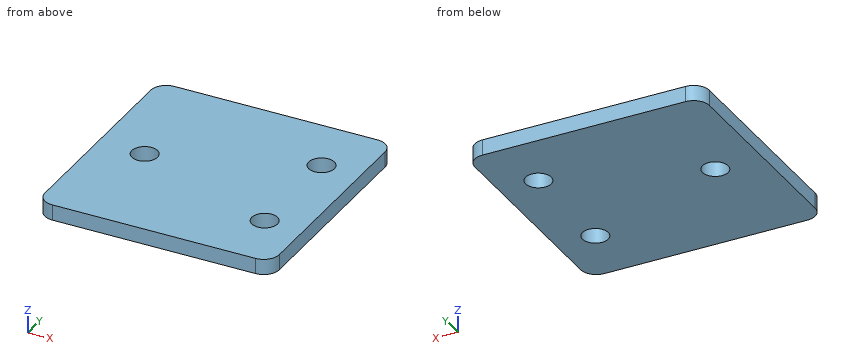
from build123d import *

# Parameters (mm, degrees)
SKETCH1_W             = 30
SKETCH1_H             = 30
BOSS_EXTRUDE1_DEPTH   = 2
FILLET1_R             = 2
F_3_0MM_DOWEL_HOLE1_D = 3.3


with BuildPart() as part:
    # Sketch1 → Boss-Extrude1 (new body)
    with BuildSketch(Plane.XY):
        Rectangle(SKETCH1_W, SKETCH1_H)
    extrude(amount=BOSS_EXTRUDE1_DEPTH)

    # Fillet1
    fillet1_edges = [part.edges().sort_by_distance(p)[0] for p in [
        (15, -15, 1),
        (-15, -15, 1),
        (-15, 15, 1),
        (15, 15, 1),
    ]]
    fillet(fillet1_edges, radius=FILLET1_R)

    # Ø3.0mm Dowel Hole1 (through all)
    with Locations(Plane(origin=(-9, 0, 2), x_dir=(1, 0, 0), z_dir=(0, 0, 1))):
        with Locations((0, 0), (19, 7), (19, -7)):
            Hole(F_3_0MM_DOWEL_HOLE1_D / 2)


solid = part.part
CAD build for the part. Positions are in the model's coordinates, mm. Coordinates: 2 decimals unless noted, no trailing zeros. Loops run counter-clockwise (first coordinate to the right, second up) from the corner with the lowest first, then second, coordinate; pieces in that order, holes last. Notation, with made-up numbers: (-37.5, -20) - (2.5, -20) arc R16 cw to (2.5, -6) - close; hole circle Ø5 at (82.25, -16.5). An arc over 180 degrees is marked (long way). Write item = value, one per line. Start each with the question number.
Q1. Drill centre lines: L1, parallel to Y at x = 10, z = 1.2; L2, parallel to Y at x = -9, z = 1; L3, parallel to X at y = 6, z = 1.1. Where is each one in solid material? Low to high.
Q2. Cut at A-A, the plane x = -9. List the corners of the cut face in (y, z).
Q3. Cut at C-C, the plane z = 1.45. List the corners of the cut face in (x, y).
Q4. Cut at B-B, the plane y = 0. List the corners of the cut face in (x, z), then the cut area to 3 significant figures.
Computed:
q1.L1 = -15 to -8.65, -5.35 to 5.35, 8.65 to 15
q1.L2 = -15 to -1.65, 1.65 to 15
q1.L3 = -15 to 8.69, 11.31 to 15
q2.outline = (-15, 0) - (-1.65, 0) - (-1.65, 2) - (-15, 2) - close; (1.65, 0) - (15, 0) - (15, 2) - (1.65, 2) - close
q3.outline = (-15, -13) arc R2 ccw to (-13, -15) - (13, -15) arc R2 ccw to (15, -13) - (15, 13) arc R2 ccw to (13, 15) - (-13, 15) arc R2 ccw to (-15, 13) - close; hole circle Ø3.3 at (-9, 0); hole circle Ø3.3 at (10, -7); hole circle Ø3.3 at (10, 7)
q4.outline = (-15, 0) - (-10.65, 0) - (-10.65, 2) - (-15, 2) - close; (-7.35, 0) - (15, 0) - (15, 2) - (-7.35, 2) - close
q4.area = 53.4 mm²
